Autodesk Inventor part; units mm, degrees
ref_plane "YZ Plane" through (0, 0, 0) normal (1, 0, 0) x (0, 1, 0)
ref_plane "XZ Plane" through (0, 0, 0) normal (0, 1, 0) x (-1, 0, 0)
ref_plane "XY Plane" through (0, 0, 0) normal (0, 0, 1) x (1, 0, 0)
sketch "Skizze1" plane through (0, 0, 0) normal (0, 1, 0) x (-1, 0, 0)
  line L0 (60.2262, 75.3938) -> (60.2262, -74.6062)
  line L1 (60.2262, -74.6062) -> (-19.7738, -60.5)
  line L2 (-19.7738, -60.5) -> (-19.7738, 61.2877)
  line L3 (-19.7738, 61.2877) -> (60.2262, 75.3938)
  arc A0 (-19.7738, 61.2877) -> (-19.7738, -60.5) centre (-8.1145, 0.3938) ccw
  circle A1 centre (-48.1145, 0) radius 1.7
  line L4 (60.2262, 60.3938) -> (20.2262, -67.5531)
  line L5 (7.0615, -65.2318) -> (-19.7534, 61.2913)
  line L6 (60.2262, 75.3938) -> (16.5507, -62.5531)
  line L7 (16.5507, -62.5531) -> (9.219, -60.2318)
  line L8 (9.219, -60.2318) -> (-14.7534, 62.1729)
  line L9 (66.5322, 80) -> (66.5322, -80)
  line L10 (66.5322, -80) -> (-19.7534, -65.5678)
  line L11 (66.5322, 80) -> (-20.7513, 65.9995)
  arc A2 (-20.7513, 65.9995) -> (-19.7534, -65.5678) centre (-7.5537, 0.3121) ccw
  point P0 (0, 0)
  point P1 (0, 0)
  dimension "d6" = 150
  dimension "d8" = 80
  dimension "d9" = 100
  dimension "d10" = 100
  dimension "d12" = 60.5
  dimension "d15" = 62
  dimension "d16" = 3.4
  dimension "d17" = 40
  dimension "d18" = 15
  dimension "d22" = 5
  dimension "d23" = 5
  dimension "d25" = 5
  dimension "d26" = 5
  dimension "d27" = 3.1473
  dimension "d28" = 7.3316
  dimension "d29" = 160
  dimension "d30" = 80
  dimension "d31" = 67
extrude "Extrusion1" add sketch "Skizze1" along normal blind 20 contours L0 L4 L1 L5 L3 L8 L7 L6 | L2 A0 | L9 L10 A2 L11
properties part number "Radaufhängung"
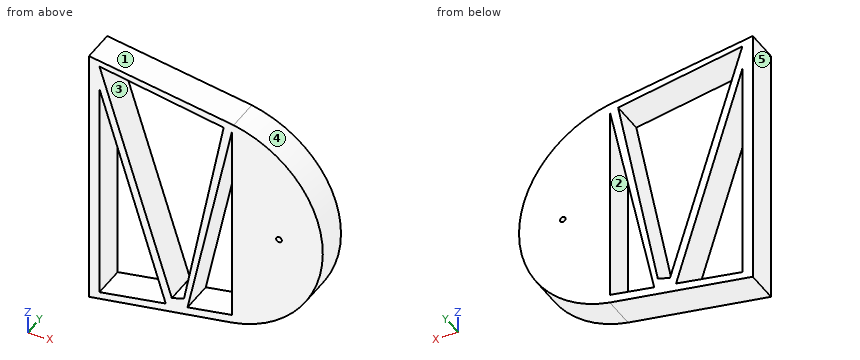
Geometry: final body of the model. Coordinates: model frame, mm. Face numbers are marked on the shaded views. A direction names the side the tool comes from. Give positions to 0.01 mm unless a question says otherwise; leave off trailing zeros. Loops run counter-clockwise (first coordinate to the right, second up) from the corner with the lowest first, then second, coordinate; pieces in that order, holes last. Notation, with made-up numbers: M -25,14.5 L 26,14.5 A16 cw 26,19.5 Z; hole C -8.75,85 d7. An arc over 180 degrees is marked long. Put each result on its own line as item: value. Start each with the question number.
1) Cut plane A-A (x = -45). Output: boundary loops of the cut face in (y, z).
2) Cut plane C-C (y = 18.25). Give the number of separate pieces and of enclosed holes in the cut face, then the cut area to 3 significant figures.
3) Access query for the marked faces 1 and 2. Directions: +Z, -Z, +X, -X, +Y, -Y. A direction counts if a zero-diameter tool reaches every point of the face in a straight line with its end or side. Return the directions, or none.
4) Ray query, line 1 along X through (y, z) = (15.75, -15.5); line 2 along X through (y, z) = (1.5, 4); line 3 along Z through (x, y) = (67, 12). Return the intervals inside material, ascending.
5) Cut plane B-B (z = 15.5). Output: boundary loops of the cut face in (x, y), then the cut area to 3 significant figures.
6) Cut plane D-D (x = 16.5). Output: boundary loops of the cut face in (y, z).
7) Contact query for flat-ended pins moving along their axis: pin 1 (10 mm diameter, centred on y = 16, z = 43, fed in from +X); pin 2 (1 mm diameter, centred on x = 18.5, y = 15, fed in from +Z); pin 3 (4 mm diameter, centred on x = -24.5, y = 10, fed in from +Z). Output: stop coordinate, or through.
8) Pull-direction query (Z, two-part tool) for the marked faces 3, 4 and 5; classes: pulls with the +Z half, pulls with the -Z half, needs draft (parallel to the pull), parting line crosses it, or undercut.
Verdict:
1. outline: M 0,-76.4 L 20,-76.4 L 20,-71.92 L 0,-71.92 Z; M 0,11.69 L 20,11.69 L 20,27.3 L 0,27.3 Z; M 0,72.71 L 20,72.71 L 20,76.55 L 0,76.55 Z
2. separate pieces: 1
2. enclosed holes: 4
2. area: 8,360 mm2
3. face 1: +Z, +X, +Y, -Y
3. face 2: +Y, -Y
4. line 1: -66.53 to -60.23, -36.5 to -31.45, -0.46 to 3.48, 19.77 to 72.66
4. line 2: -66.53 to -60.23, -42.6 to -37.62, 3.36 to 7.61, 19.77 to 74.45
4. line 3: -30.59 to 31.22
5. outline: M -66.53,0 L -60.23,0 L -60.23,20 L -66.53,20 Z; M -46.19,0 L -41.26,0 L -41.26,20 L -46.19,20 Z; M 5.61,0 L 10.05,0 L 10.05,20 L 5.61,20 Z; M 19.77,0 L 72.81,0 L 72.81,20 L 19.77,20 Z
5. area: 1,370 mm2
6. outline: M 0,-66.11 L 20,-66.11 L 20,-61.08 L 0,-61.08 Z; M 0,45.94 L 20,45.94 L 20,66.68 L 0,66.68 Z
7. pin 1: x = 62.95
7. pin 2: z = 66.44
7. pin 3: z = 73.58
8. face 3: undercut
8. face 4: parting line crosses it
8. face 5: needs draft
